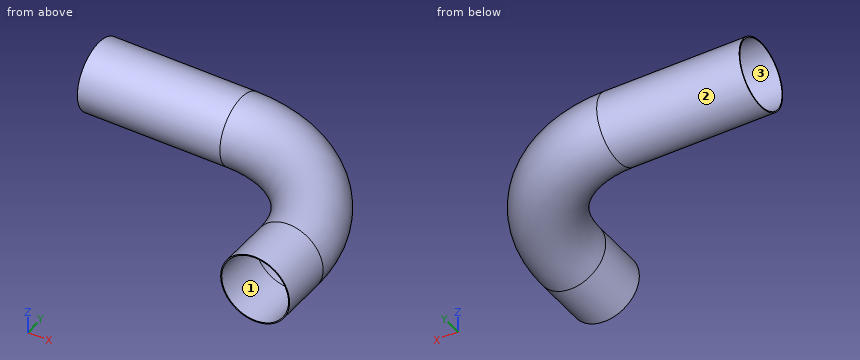
from build123d import *

# Parameters (mm, degrees)
SKETCH2_R = 13.5
SKETCH3_R = 13.1


with BuildPart() as part:
    # Sweep1: sweep along a path in Sketch1
    with BuildLine(Plane.XY) as sweep1_path:
        Line((0, 0), (55.82246027, 0))
        ThreePointArc((55.82246027, 0), (91.17779933, -14.644660941), (105.82246027, -50))
        Line((105.82246027, -50), (105.82246027, -70.851970701))
    # Sketch2 → Sweep1 (sweep)
    with BuildSketch(Plane(origin=(0, 0, 0), x_dir=(0, 0, -1), z_dir=(1, 0, 0))):
        Circle(SKETCH2_R)
    sweep(path=sweep1_path.line)

    # Cut-Sweep1: sweep along a path in Sketch1<2>
    with BuildLine(Plane.XY) as cut_sweep1_path:
        Line((0, 0), (55.82246027, 0))
        ThreePointArc((55.82246027, 0), (91.17779933, -14.644660941), (105.82246027, -50))
        Line((105.82246027, -50), (105.82246027, -70.851970701))
    # Sketch3 → Cut-Sweep1 (sweep, cut)
    with BuildSketch(Plane.ZY):
        Circle(SKETCH3_R)
    sweep(path=cut_sweep1_path.line, mode=Mode.SUBTRACT)


solid = part.part
Design review of the part built by this model. Coordinates are the model's own, in mm. Face numbers are marked on the shaded views. Round coordinates to 2 decimals unless told otherwise and drop trailing zeros. Write each loop counter-clockwise with the first axis right and the second up, starting at its lowest first coordinate (ties: lowest second). Pieces come first, ordered by that corner, then holes.
Item 1: Draft analysis for pull direction Y (two halves, no side actions). For the marked faces 1, 2 and 3, state which applies: released by +Y, released by -Y, zero draft, split by the parting line, or undercut.
Item 2: Wall thickness on L1, parallel to X at y = -56.75, z = 0; L2, parallel to Y at x = 18.5, z = 0; L3, parallel to Y at x = 65.5, z = -0.75: over which ranges is each line inside the solid? List them lowest first.
Item 3: Consider section A-A on z = 0. Give the boundary of the cut face in (x, y), and give its area (3 significant figures).
Item 4: Consider section B-B on x = 28.5. Give the boundary of the cut face in (y, z), and give its area (3 significant figures).
Item 5: For pin 1 Ø1.5 at (y, z) = (-17.5, -1.5) entering from +X; pin 2 Ø1 at (x, z) = (26, 7) entering from +Y; pin 3 Ø3 at (y, z) = (-3, -1) entering from -X, all flat-tipped, find the tip position at first contact; note any pin that passes through.
Item 6: Consider section C-C on z = -11. Give the boundary of the cut face in (x, y).
Check values:
1. face 1: zero draft
1. face 2: split by the parting line
1. face 3: undercut
2. L1: x = 92.32 to 92.72, 118.92 to 119.32
2. L2: y = -13.5 to -13.1, 13.1 to 13.5
2. L3: y = -14.78 to -14.37, 12.33 to 12.74
3. outline: (0, -13.5) - (55.82, -13.5) arc R36.5 cw to (92.32, -50) - (92.32, -70.85) - (92.72, -70.85) - (92.72, -50) arc R36.9 ccw to (55.82, -13.1) - (0, -13.1) - close; (0, 13.1) - (55.82, 13.1) arc R63.1 cw to (118.92, -50) - (118.92, -70.85) - (119.32, -70.85) - (119.32, -50) arc R63.5 ccw to (55.82, 13.5) - (0, 13.5) - close
3. area: 124 mm2
4. outline: circle Ø27 at (0, 0); hole circle Ø26.2 at (0, 0)
4. area: 33.4 mm2
5. pin 1: stops at x = 110.73
5. pin 2: stops at y = 11.83
5. pin 3: stops at x = 96.12
6. outline: (0, -7.83) - (55.82, -7.83) arc R42.17 cw to (98, -50) - (98, -70.85) - (98.71, -70.85) - (98.71, -50) arc R42.89 ccw to (55.82, -7.11) - (0, -7.11) - close; (0, 7.11) - (55.82, 7.11) arc R57.11 cw to (112.94, -50) - (112.94, -70.85) - (113.65, -70.85) - (113.65, -50) arc R57.83 ccw to (55.82, 7.83) - (0, 7.83) - close
